```python
from build123d import *

# Parameters (mm, degrees)
F0_W         = 18
F0_H         = 18
F1_DEPTH     = 18
F2_W         = 10
F2_H         = 10
F2_W_2       = 3
F2_H_2       = 3
F3_DEPTH     = 5
F4_DEPTH     = 8
F5_R         = 2
F6_R         = 2
F7_T1_DEPTH  = 8
F7_T3_DEPTH  = 8
F7_T5_DEPTH  = 8
F7_S9_W      = 2
F7_S9_H      = 2
F7_T10_DEPTH = 2
F7_S15_W     = 2
F7_S15_H     = 2
F7_T16_DEPTH = 2
F7_S21_W     = 2
F7_S21_H     = 2
F7_T22_DEPTH = 2
F8_R         = 2
F10_DEPTH    = 20
F12_DEPTH    = 20


# Not quite as in the source:
# - a fillet or chamfer that OpenCascade refuses, or shapes differently, is made with other operations: its cross-section is extruded or revolved along the edge and cut away or added


with BuildPart() as f1:
    # F0 (on Front) → F1 (new body)
    with BuildSketch(Plane.XZ):
        with Locations((-9, 9)):
            Rectangle(F0_W, F0_H)
    extrude(amount=-F1_DEPTH)

    # F2 (on Top) → F3 (join)
    with BuildSketch(Plane.XY):
        Rectangle(F2_W, F2_H)
        with Locations((-6.5, 0)):
            Rectangle(F2_W_2, F2_H)
        with Locations((0, 6.5)):
            Rectangle(F2_W, F2_H_2)
        with Locations((-6.5, 6.5)):
            Rectangle(F2_W_2, F2_H_2)
    extrude(amount=-F3_DEPTH)

    # F2 (on Top) → F4 (join)
    with BuildSketch(Plane.XY):
        Rectangle(F2_W, F2_H)
        with Locations((-6.5, 0)):
            Rectangle(F2_W_2, F2_H)
        with Locations((0, 6.5)):
            Rectangle(F2_W, F2_H_2)
        with Locations((-6.5, 6.5)):
            Rectangle(F2_W_2, F2_H_2)
    extrude(amount=F4_DEPTH)

    # F5
    f5_edges = [f1.edges().sort_by_distance(p)[0] for p in [
        (-18, 18, 9),
        (-18, 9, 18),
        (-9, 18, 18),
    ]]
    fillet(f5_edges, radius=F5_R)

    # F6
    f6_edges = [f1.edges().sort_by_distance(p)[0] for p in [
        (0, 8, 18),
        (-8, 0, 18),
        (-18, 8, 0),
    ]]
    fillet(f6_edges, radius=F6_R)

    # F7: fillet of radius 2 on 3 edges, made by hand

    # F7_s2 → F7_t1 (cut)
    with BuildSketch(Plane.XZ.offset(-16)):
        with BuildLine():
            ThreePointArc((-2, 0), (-0.5857864376, 0.5857864376), (0, 2))
            Line((0, 2), (0, 0))
            Line((0, 0), (-2, 0))
        make_face()
    extrude(amount=F7_T1_DEPTH, mode=Mode.SUBTRACT)

    # F7_s4 → F7_t3 (cut)
    with BuildSketch(Plane.XY.offset(8)):
        with BuildLine():
            ThreePointArc((0, 2), (-0.5857864376, 0.5857864376), (-2, 0))
            Line((-2, 0), (0, 0))
            Line((0, 0), (0, 2))
        make_face()
    extrude(amount=F7_T3_DEPTH, mode=Mode.SUBTRACT)

    # F7_s6 → F7_t5 (cut)
    with BuildSketch(Plane.YZ.offset(-16)):
        with BuildLine():
            ThreePointArc((2, 0), (0.5857864376, 0.5857864376), (0, 2))
            Line((0, 2), (0, 0))
            Line((0, 0), (2, 0))
        make_face()
    extrude(amount=F7_T5_DEPTH, mode=Mode.SUBTRACT)


with BuildPart() as f7_tool8:
    # F7_s9 → F7_t10 (new body)
    with BuildSketch(Plane.XY.offset(2)):
        with Locations((-17, 1)):
            Rectangle(F7_S9_W, F7_S9_H)
    extrude(amount=-F7_T10_DEPTH)

    # F7_s11 → F7_t12 (revolve, cut)
    with BuildSketch(Plane(origin=(-16, 2, 2), x_dir=(0.7071067812, 0.7071067812, 0), z_dir=(-0.7071067812, 0.7071067812, 0))):
        with BuildLine():
            ThreePointArc((0, -2), (2, 0), (0, 2))
            Line((0, 2), (0, -2))
        make_face()
    revolve(axis=Axis((-16, 2, 2), (0, 0, -1)), mode=Mode.SUBTRACT)


with BuildPart() as f1_1:
    add(f1.part)

    # F7_t7: cut F7_tool8
    add(f7_tool8.part, mode=Mode.SUBTRACT)


with BuildPart() as f7_tool14:
    # F7_s15 → F7_t16 (new body)
    with BuildSketch(Plane.YZ.offset(-2)):
        with Locations((1, 17)):
            Rectangle(F7_S15_W, F7_S15_H)
    extrude(amount=F7_T16_DEPTH)

    # F7_s17 → F7_t18 (revolve, cut)
    with BuildSketch(Plane(origin=(-2, 2, 16), x_dir=(0, 0.7071067812, -0.7071067812), z_dir=(0, -0.7071067812, -0.7071067812))):
        with BuildLine():
            ThreePointArc((0, -2), (2, 0), (0, 2))
            Line((0, 2), (0, -2))
        make_face()
    revolve(axis=Axis((-2, 2, 16), (1, 0, 0)), mode=Mode.SUBTRACT)


with BuildPart() as f1_2:
    add(f1_1.part)

    # F7_t13: cut F7_tool14
    add(f7_tool14.part, mode=Mode.SUBTRACT)


with BuildPart() as f7_tool20:
    # F7_s21 → F7_t22 (new body)
    with BuildSketch(Plane.XY.offset(2)):
        with Locations((-1, 17)):
            Rectangle(F7_S21_W, F7_S21_H)
    extrude(amount=-F7_T22_DEPTH)

    # F7_s23 → F7_t24 (revolve, cut)
    with BuildSketch(Plane(origin=(-2, 16, 2), x_dir=(-0.7071067812, -0.7071067812, 0), z_dir=(0.7071067812, -0.7071067812, 0))):
        with BuildLine():
            ThreePointArc((0, -2), (2, 0), (0, 2))
            Line((0, 2), (0, -2))
        make_face()
    revolve(axis=Axis((-2, 16, 2), (0, 0, -1)), mode=Mode.SUBTRACT)


with BuildPart() as f1_3:
    add(f1_2.part)

    # F7_t19: cut F7_tool20
    add(f7_tool20.part, mode=Mode.SUBTRACT)

    # F8
    f8_edges = [f1_3.edges().sort_by_distance(p)[0] for p in [
        (-8, -2.5, 8),
        (2.5, 8, 8),
        (-8, 8, -2.5),
    ]]
    fillet(f8_edges, radius=F8_R)

    # F9 (on Front) → F10 (cut, symmetric)
    with BuildSketch(Plane.XZ):
        Polygon((5, -5), (-18, 18), (-18, -5), align=None)
    extrude(amount=F10_DEPTH, both=True, mode=Mode.SUBTRACT)

    # F11 (on Right) → F12 (cut, symmetric)
    with BuildSketch(Plane.YZ):
        Polygon((18, 18), (-5, -5), (18, -5), align=None)
    extrude(amount=F12_DEPTH, both=True, mode=Mode.SUBTRACT)


solid = f1_3.part
```
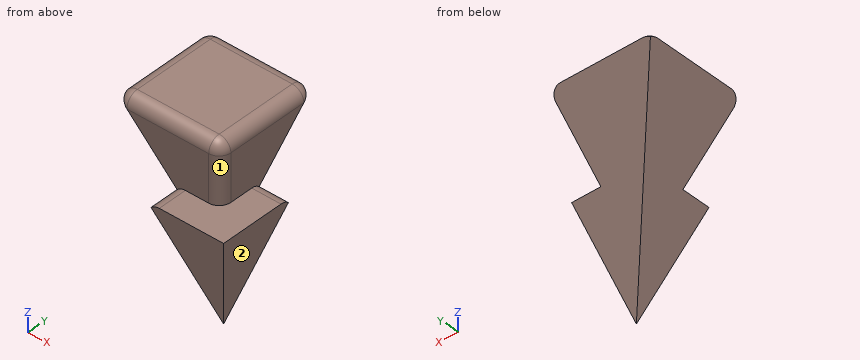
Could you check a few things on this model? Use its own coordinates, in mm. Face numbers are marked on the shaded views. A direction names the side the tool comes from. Give positions to 0.01 mm unless a question says otherwise; leave off trailing zeros. Order: outer loops, then holes, each group sorted by start corner. A loop starts at its lowest first (then second) coordinate and runs counter-clockwise, first axis right, second up.
Q1. Suppose I cut it at B-B, the plane x = 3. Write out the boundary of the cut face in (y, z), and give its area (3 significant figures).
Q2. For the marked faces 1 and 2, which set-ups out of +Z, -Z, +X, -X, +Y, -Y let a thin tool reach every point of the face, with its end or its side?
Q3. If I drill on line 1 along Y through (x, z) = (3, 6); line 2 along Z through (x, y) = (-9, 16); line 3 along X through (y, z) = (-3, 1), over which ranges is the centre line in solid material (lowest first)?
Q4. I'm going to push flat-ended pins straight in: P1, Ø12, axis at x = 0.5, z = 5, coming from the +Y side; P2, Ø6, axis at x = -0.5, y = -2.5, coming from the -Z side; P3, Ø2.5, axis at x = -12, z = 9.5, coming from the -Y side; P4, Ø4, axis at x = 1, z = 8, coming from the +Y side. Where does each tip first touch, or does it pass through?
Q5. Suppose I cut it at C-C, the plane z = -2.5. Write out the boundary of the cut face in (x, y).
Q6. Suppose I cut it at D-D, the plane y = 8.25. Write out the boundary of the cut face in (x, z), and give its area (3 significant figures).
Q7. Suppose I cut it at A-A, the plane y = 14. Write out the boundary of the cut face in (x, z), and give its area (3 significant figures).
Solution:
1. outline: (-5, -3) - (-3, -3) - (7.41, 7.41) arc R2 ccw to (6, 8) - (-5, 8) - close
1. area: 82.1 mm2
2. face 1: +Z, +X, -Y
2. face 2: +Z, -Z, +X, +Y, -Y
3. line 1: y = -5 to 6
3. line 2: z = 16 to 18
3. line 3: x = -1 to 5
4. P1: stops at y = 10.98
4. P2: stops at z = -2.5
4. P3: passes through
4. P4: stops at y = 9.73
5. outline: (2.5, -5) - (5, -5) - (5, -2.5) - (2.5, -2.5) - close
6. outline: (-17.41, 17.41) - (-8.25, 8.25) - (0, 8.25) - (0, 16) arc R2 ccw to (-2, 18) - (-16, 18) arc R2 ccw to start
6. area: 127 mm2
7. outline: (-17.41, 17.41) - (-14, 14) - (0, 14) - (0, 16) arc R2 ccw to (-2, 18) - (-16, 18) arc R2 ccw to start
7. area: 62.7 mm2
